```python
from build123d import *

# Parameters (mm, degrees)
SKETCH1_W               = 330.2
SKETCH1_H               = 12.7
SKETCH1_R               = 3.429
EXTRUDE1_DEPTH          = 1.5875
CUT_EXTRUDE2_DEPTH      = 7.35
CUT_EXTRUDE2_DEPTH_BACK = 7.35


with BuildPart() as part:
    # Sketch1 → Extrude1 (new body)
    with BuildSketch(Plane(origin=(0, 0, 0), x_dir=(1, 0, 0), z_dir=(0, 1, 0))):
        with Locations((165.1, 0)):
            Rectangle(SKETCH1_W, SKETCH1_H)
        with Locations(Location((320.675, 0, 0), (0, 0, 270))):  # turned: the seam where the file's is
            Circle(SKETCH1_R, mode=Mode.SUBTRACT)
    extrude(amount=EXTRUDE1_DEPTH)

    # Sketch2 → Cut-Extrude2 (cut, two sides)
    with BuildSketch(Plane.XY) as cut_extrude2_sk:
        Polygon((330.2, 0), (330.2, 2.264018557), (301.954487886, 2.264018557), align=None)
    extrude(amount=CUT_EXTRUDE2_DEPTH, mode=Mode.SUBTRACT)
    extrude(cut_extrude2_sk.sketch, amount=-CUT_EXTRUDE2_DEPTH_BACK, mode=Mode.SUBTRACT)


solid = part.part
```
CAD build for the part. Positions are in the model's coordinates, mm. Round coordinates to 2 decimals unless told otherwise and drop trailing zeros. Loops run counter-clockwise (first coordinate to the right, second up) from the corner with the lowest first, then second, coordinate; pieces in that order, holes last. Notation, with made-up numbers: M 55,85.5 L 76,85.5 A27 cw 76,101.5 Z; hole C 57,0.5 d7. An arc over 180 degrees is marked long. Use a Markdown table: item, result. Add a question column.
(1) Cut at A-A (z = 0). Give the cut face in (x, y).
(2) Drill centre line: line 1 (X direction, y = 0.9, z = 1.75). Where is it in solid material? Low to high.
(3) Pull direction X, two halves, no side cores. Call faces 1 (the face through (317.328, 0.397, -0.743)), 2 (the face through (317.96, 0.98, 2.73)), 3 (the face through (163, 0, 0)): +X half, -X half, draft (parallel to the pull), parting line (faces both ways), or undercut.
Geometry says:
| question | item | result |
|---|---|---|
| 1 | outline | M 0,0 L 317.25,0 L 317.25,1.04 L 310.39,1.59 L 0,1.59 Z; M 324.1,0 L 330.2,0 L 324.1,0.49 Z |
| 2 | line 1 | x = 0 to 317.73 |
| 3 | face 1 | undercut |
| 3 | face 2 | +X half |
| 3 | face 3 | draft |
